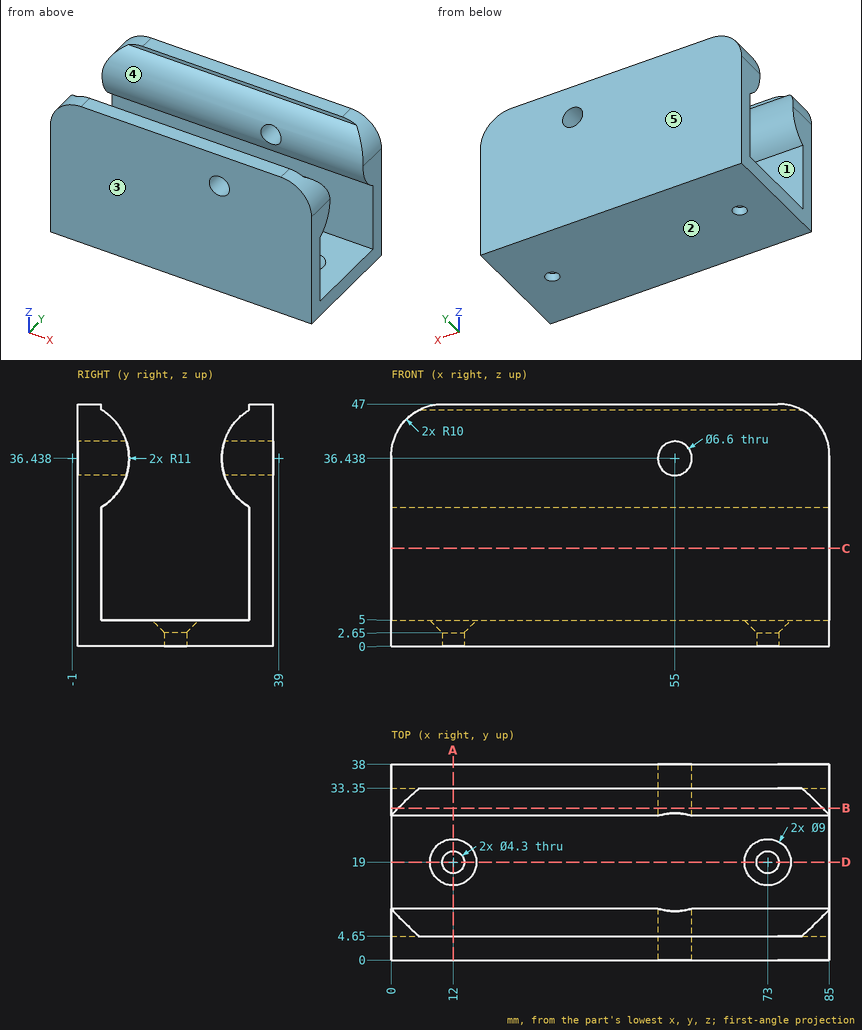
Study the drawing (mm; zero at the part's minimum x, y, z) and answer. A direction names the side the tool comes from. Round coordinates to 2 decimals unless told otherwise and drop trailing zeros. Order: outer loops, then holes, each group sorted by start corner. A loop starts at its lowest first (then second) coordinate and runs counter-clockwise, first axis right, second up. Notation, with made-up numbers: (80, 84.5) -> (131, 84.5) arc R19 cw to (131, 88.5) -> close; hole circle Ø1 at (61, 26.25). An arc over 180 degrees is marked (long way). Answer as CSV lines item,"result". Start each with the question number.
(1) Flat-ended cylindrical pins translate along their axes: pin 1 Ø4 at (x, z) = (55, 36.44) entering from -Y; pin 2 Ø14.5 at (x, y) = (59, 20) entering from +Z; pin 3 Ø5 at (x, y) = (73, 19) entering from +Z; pin 4 Ø4 at (x, y) = (33.5, 32) entering from -Z. Find the tip coordinate at first contact, or state that the pin passes through.
(2) The part is cut by section B-B (y = 29.5). Determine the outline of the cut face in (x, z), then the cut area to 3 significant figures.
(3) Find the intervals of material crossed by probe 1 along Z at (x, y) = (55, 36); probe 2 along Y at (x, z) = (55, 15); probe 3 along Y at (x, z) = (73, 2.15), in increasing order. Write a range as from..to.
(4) The part is cut by section C-C (z = 19). Determine the outline of the cut face in (x, y).
(5) The part is cut by section A-A (x = 12). Determine the outline of the cut face in (y, z).
(6) A tool of negligible diameter and unlimited length cuts with its end or side. For the marked faces 4 and 5, from which of +Z, -Z, +X, -X, +Y, -Y can it reach the whole face along a straight path? Write none if from no direction.
(7) For a pull along Y with two mould halves and no side action, classify the marked faces 1, 2 and 3 as +Y half, -Y half, draft (parallel to the pull), parting line (faces both ways), or undercut.
(8) The part is cut by section D-D (y = 19). Determine the outline of the cut face in (x, z), then the cut area to 3 significant figures.
Evaluation:
1,pin 1,"through"
1,pin 2,"z = 5"
1,pin 3,"z = 3"
1,pin 4,"z = 0"
2,outline,"(0, 0) -> (85, 0) -> (85, 5) -> (0, 5) -> close; (0, 30.89) -> (85, 30.89) -> (85, 37) arc R10 ccw to (83.67, 41.98) -> (1.33, 41.98) arc R10 ccw to (0, 37) -> close; hole circle Ø6.6 at (55, 36.44)"
2,area,"1,330 mm²"
3,probe 1,"0..33.14, 39.74..47"
3,probe 2,"0..4.65, 33.35..38"
3,probe 3,"0..16.85, 21.15..38"
4,outline,"(0, 0) -> (85, 0) -> (85, 4.65) -> (0, 4.65) -> close; (0, 33.35) -> (85, 33.35) -> (85, 38) -> (0, 38) -> close"
5,outline,"(0, 0) -> (16.85, 0) -> (16.85, 2.65) -> (14.5, 5) -> (4.65, 5) -> (4.65, 27) arc R11 ccw to (4.65, 45.88) -> (4.65, 47) -> (0, 47) -> close; (21.15, 0) -> (38, 0) -> (38, 47) -> (33.35, 47) -> (33.35, 45.88) arc R11 ccw to (33.35, 27) -> (33.35, 5) -> (23.5, 5) -> (21.15, 2.65) -> close"
6,face 4,"+X, -X"
6,face 5,"+Z, -Z, +X, -X, +Y"
7,face 1,"undercut"
7,face 2,"draft"
7,face 3,"-Y half"
8,outline,"(0, 0) -> (9.85, 0) -> (9.85, 2.65) -> (7.5, 5) -> (0, 5) -> close; (14.15, 0) -> (70.85, 0) -> (70.85, 2.65) -> (68.5, 5) -> (16.5, 5) -> (14.15, 2.65) -> close; (75.15, 0) -> (85, 0) -> (85, 5) -> (77.5, 5) -> (75.15, 2.65) -> close"
8,area,"371 mm²"
